```python
from build123d import *

# Parameters (mm, degrees)
SKETCH1_W           = 500
SKETCH1_H           = 200
BOSS_EXTRUDE1_DEPTH = 18
SKETCH2_R           = 4
CUT_EXTRUDE1_DEPTH  = 10
CUT_EXTRUDE2_DEPTH  = 30


with BuildPart() as part:
    # Sketch1 → Boss-Extrude1 (new body)
    with BuildSketch(Plane(origin=(0, 0, 0), x_dir=(1, 0, 0), z_dir=(0, 1, 0))):
        with Locations((250, 100)):
            Rectangle(SKETCH1_W, SKETCH1_H)
    extrude(amount=BOSS_EXTRUDE1_DEPTH)

    # Sketch2 → Cut-Extrude1 (cut)
    with BuildSketch(Plane(origin=(0, 18, 0), x_dir=(1, 0, 0), z_dir=(0, 1, 0))):
        with Locations(Location((9, 180, 0), (0, 0, 270))):
            Circle(SKETCH2_R)
        with Locations(Location((9, 148, 0), (0, 0, 270))):
            Circle(SKETCH2_R)
        with Locations(Location((9, 116, 0), (0, 0, 270))):
            Circle(SKETCH2_R)
        with Locations(Location((9, 84, 0), (0, 0, 270))):
            Circle(SKETCH2_R)
        with Locations(Location((9, 52, 0), (0, 0, 270))):
            Circle(SKETCH2_R)
        with Locations(Location((9, 20, 0), (0, 0, 270))):
            Circle(SKETCH2_R)
        with Locations(Location((491, 20, 0), (0, 0, 90))):
            Circle(SKETCH2_R)
        with Locations(Location((491, 52, 0), (0, 0, 90))):
            Circle(SKETCH2_R)
        with Locations(Location((491, 84, 0), (0, 0, 90))):
            Circle(SKETCH2_R)
        with Locations(Location((491, 116, 0), (0, 0, 90))):
            Circle(SKETCH2_R)
        with Locations(Location((491, 148, 0), (0, 0, 90))):
            Circle(SKETCH2_R)
        with Locations(Location((491, 180, 0), (0, 0, 90))):
            Circle(SKETCH2_R)
    extrude(amount=-CUT_EXTRUDE1_DEPTH, mode=Mode.SUBTRACT)

    # Sketch3 → Cut-Extrude2 (cut)
    with BuildSketch(Plane(origin=(0, 18, 0), x_dir=(1, 0, 0), z_dir=(0, 1, 0))):
        with BuildLine():
            Line((160, 150), (340, 150))
            ThreePointArc((340, 150), (347.071067812, 147.071067812), (350, 140))
            Line((350, 140), (350, 60))
            ThreePointArc((350, 60), (347.071067812, 52.928932188), (340, 50))
            Line((340, 50), (160, 50))
            ThreePointArc((160, 50), (152.928932188, 52.928932188), (150, 60))
            Line((150, 60), (150, 140))
            ThreePointArc((150, 140), (152.928932188, 147.071067812), (160, 150))
        make_face()
    extrude(amount=-CUT_EXTRUDE2_DEPTH, mode=Mode.SUBTRACT)


solid = part.part
```
Input: part model. Units: mm. Frame: model coordinates. A direction names the side the tool comes from. Give positions to 0.01 mm unless a question says otherwise; leave off trailing zeros. Order: outer loops, then holes, each group sorted by start corner. A loop starts at its lowest first (then second) coordinate and runs counter-clockwise, first axis right, second up. Notation, with made-up numbers: (48.25, 6) - (107.25, 6) arc R20 ccw to (107.25, 24) - close; hole circle Ø6 at (-7, 18.5). An arc over 180 degrees is marked (long way). Use a Markdown table: item, result.
(1) Pin query (flat end, axial travel): pin 1 (2.5 mm diameter, centred on x = 490, z = -51.5, fed in from +Y). Return the tip coordinate at first contact, or that it passes through.
Computed values:
| item | result |
|---|---|
| pin 1 | stops at y = 8 |
(2) Section query B-B (z = -130.5). Output: boundary loops of the cut face in (x, y).
Computed values:
| item | result |
|---|---|
| outline | (0, 0) - (150, 0) - (150, 18) - (0, 18) - close; (350, 0) - (500, 0) - (500, 18) - (350, 18) - close |
(3) Line query: line 1 (X direction, y = 11.5, z = -180); line 2 (Z direction, x = 191, y = 6.5); line 3 (X direction, y = 12.25, z = -139). Output: solid intervals per line, ascending. Write a range as from..to.
Computed values:
| item | result |
|---|---|
| line 1 | x = 0..5, 13..487, 495..500 |
| line 2 | z = -200..-150, -50..0 |
| line 3 | x = 0..150, 350..500 |
(4) Section query C-C (y = 3.25). Output: boundary loops of the cut face in (x, z).
Computed values:
| item | result |
|---|---|
| outline | (0, -200) - (500, -200) - (500, 0) - (0, 0) - close; hole (150, -140) arc R10 ccw to (160, -150) - (340, -150) arc R10 ccw to (350, -140) - (350, -60) arc R10 ccw to (340, -50) - (160, -50) arc R10 ccw to (150, -60) - close |
(5) Draft query along X for faces 3 (the flat face through (247, 9, 0)), 4 (the flat face through (251, 9, -50)), 5 (the flat face through (500, 9, -99)), 6 (the flat face through (0, 9, -99)). Return one class per face: released by +X, released by -X, zero draft, split by the parting line, or undercut.
Computed values:
| item | result |
|---|---|
| face 3 | zero draft |
| face 4 | undercut |
| face 5 | released by +X |
| face 6 | released by -X |
(6) Section query A-A (x = 231.5). Output: boundary loops of the cut face in (y, z).
Computed values:
| item | result |
|---|---|
| outline | (0, -200) - (18, -200) - (18, -150) - (0, -150) - close; (0, -50) - (18, -50) - (18, 0) - (0, 0) - close |
(7) Access query for faces 1 (the flat face through (247, 0, -35)), 2 (the cylindrical face through (152.85, 9.13, -146.99)). Directions: +Z, -Z, +X, -X, +Y, -Y. A direction counts if a zero-diameter tool reaches every point of the face in a straight line with its end or side. Return the directions, or none.
Computed values:
| item | result |
|---|---|
| face 1 | +Z, -Z, +X, -X, -Y |
| face 2 | +Y, -Y |
